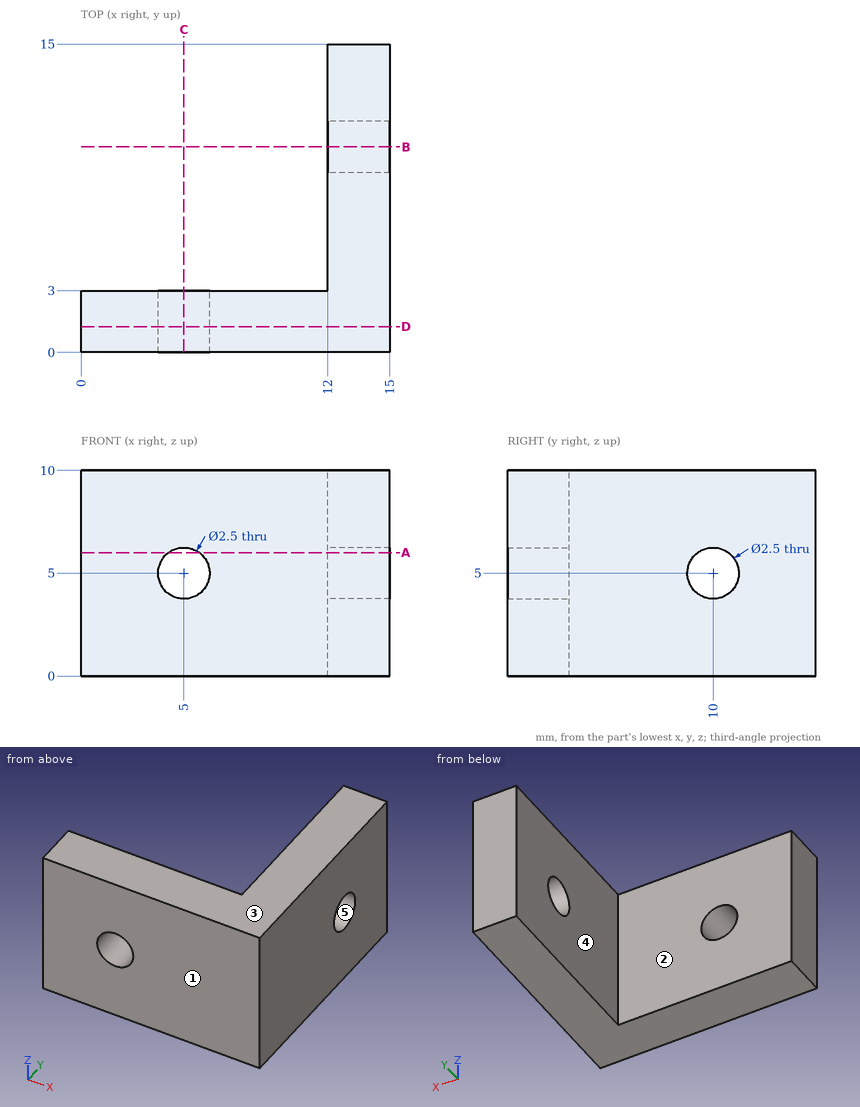
For this review, use the dimensioned drawing (mm, ordinates from the lowest corner) and the shaded views. A direction names the side the tool comes from. Round coordinates to 2 decimals unless told otherwise and drop trailing zeros. Loops run counter-clockwise (first coordinate to the right, second up) from the corner with the lowest first, then second, coordinate; pieces in that order, holes last. Notation, with made-up numbers: M -34.75,61.25 L -24.75,61.25 A16 cw -24.75,73.25 Z; hole C -27,21 d2. An arc over 180 degrees is marked long. Answer as CSV lines item,"result".
1. To check wall thickness, follow L1, parallel to Z at x = 5, y = 2; L2, parallel to Y at x = 12.75, z = 5; L3, parallel to X at y = 1.2, z = 5. State the ranges of each line that lie inside material, in increasing order. Write a range as [from, to].
Outcome:
L1,"z = [0, 3.75], [6.25, 10]"
L2,"y = [0, 8.75], [11.25, 15]"
L3,"x = [0, 3.75], [6.25, 15]"
2. We need section A-A (z = 6). Give the boundary of the cut face in (x, y).
Outcome:
outline,"M 0,0 L 4.25,0 L 4.25,3 L 0,3 Z; M 5.75,0 L 15,0 L 15,9.25 L 12,9.25 L 12,3 L 5.75,3 Z; M 12,10.75 L 15,10.75 L 15,15 L 12,15 Z"
3. We need section C-C (x = 5). Give the boundary of the cut face in (y, z).
Outcome:
outline,"M 0,0 L 3,0 L 3,3.75 L 0,3.75 Z; M 0,6.25 L 3,6.25 L 3,10 L 0,10 Z"
4. For the marked faces 1 and 2, list the 3-axis set-ups (+Z, -Z, +X, -X, +Y, -Y) from which the entire face can be reached by the end or side of a thin tool; tool diameter is ignored.
Outcome:
face 1,"+Z, -Z, +X, -X, -Y"
face 2,"+Z, -Z, -X, +Y"
5. Insertion check: pin 1 Ø5 at (y, z) = (7.5, 6) entering from -X; pin 2 Ø3 at (x, z) = (5, 5) entering from +Y. Each pin has a flat end and moves straight along its axis. Give the tip position at first contact, or say it passes through.
Outcome:
pin 1,"stops at x = 12"
pin 2,"stops at y = 3"
6. We need section B-B (y = 10). Give the boundary of the cut face in (x, z), plus the area to 3 significant figures.
Outcome:
outline,"M 12,0 L 15,0 L 15,3.75 L 12,3.75 Z; M 12,6.25 L 15,6.25 L 15,10 L 12,10 Z"
area,"22.5 mm2"
7. Draft analysis for pull direction Z (two halves, no side actions). For the marked faces 3, 4 and 5, state which applies: pulls with the +Z half, pulls with the -Z half, needs draft (parallel to the pull), parting line crosses it, or undercut.
Outcome:
face 3,"pulls with the +Z half"
face 4,"needs draft"
face 5,"undercut"
8. We need section D-D (y = 1.25). Give the boundary of the cut face in (x, z).
Outcome:
outline,"M 0,0 L 15,0 L 15,10 L 0,10 Z; hole C 5,5 d2.5"
